from build123d import *

# Parameters (mm, degrees)
F0_W     = 13.3
F0_H     = 13.3
F0_W_2   = 13.4
F0_H_2   = 13.4
F0_W_3   = 13.5
F0_H_3   = 13.5
F0_W_4   = 13.6
F0_H_4   = 13.6
F1_DEPTH = 5


with BuildPart() as f1:
    # F0 (on Top) → F1 (new body)
    with BuildSketch(Plane.XY):
        Polygon((27.294878, 11.65), (-52.963719, 11.65), (-52.963719, -11.65), (30.85, -11.65), (30.85, 8.722694), align=None)
        with Locations((-41.313719, 0)):
            Rectangle(F0_W, F0_H, mode=Mode.SUBTRACT)
        with Locations((-19.05, 0)):
            Rectangle(F0_W_2, F0_H_2, mode=Mode.SUBTRACT)
        Rectangle(F0_W_3, F0_H_3, mode=Mode.SUBTRACT)
        with Locations((19.05, 0)):
            Rectangle(F0_W_4, F0_H_4, mode=Mode.SUBTRACT)
    extrude(amount=F1_DEPTH)


solid = f1.part
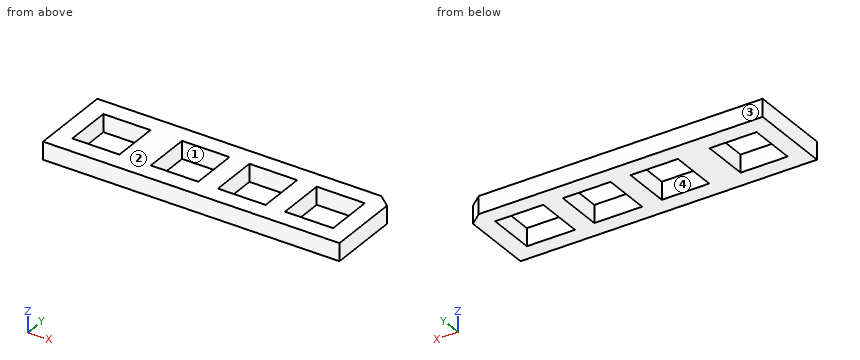
Build history of the part. All positions in model axes, mm. Face numbers are marked on the shaded views. A direction names the side the tool comes from. Round coordinates to 2 decimals unless told otherwise and drop trailing zeros. Loops run counter-clockwise (first coordinate to the right, second up) from the corner with the lowest first, then second, coordinate; pieces in that order, holes last. Notation, with made-up numbers: (-3, 75) -> (34, 75) arc R10 ccw to (34, 94) -> close; hole circle Ø10 at (46, 77.5). An arc over 180 degrees is marked (long way). One line per item, written item: value. Start each with the question number.
Q1. Probe line 1 along X through (y, z) = (-6, 3.3); line 2 along Y through (x, z) = (-19, 4.45); line 3 along Y through (x, z) = (-43, 0.4). List the from-to ranges inside material, lowest first.
Q2. 3-axis set-ups, long thin cutter, end or side, ignore diameter. For the marked faces 1 and 2: which of +Z, -Z, +X, -X, +Y, -Y reach the whole face in a straight line?
Q3. Cut at A-A on x = 23. List the corners of the cut face in (y, z), plus the area to 3 significant figures.
Q4. Cut at B-B on y = 2.75. List the corners of the cut face in (x, z), plus the area to 3 significant figures.
Q5. Two-plate mould, pull along X, no slides. Class the marked faces 3 and 4: released by +X, released by -X, zero draft, split by the parting line, or undercut.
Q6. Cut at C-C on z = 0.95. List the corners of the cut face in (x, y).
Q7. Cut at D-D on x = -18.5. List the corners of the cut face in (y, z).
Computed:
1. line 1: -52.96 to -47.96, -34.66 to -25.75, -12.35 to -6.75, 6.75 to 12.25, 25.85 to 30.85
1. line 2: -11.65 to -6.7, 6.7 to 11.65
1. line 3: -11.65 to -6.65, 6.65 to 11.65
2. face 1: +Z, -Z
2. face 2: +Z, +X, -X, +Y, -Y
3. outline: (-11.65, 0) -> (-6.8, 0) -> (-6.8, 5) -> (-11.65, 5) -> close; (6.8, 0) -> (11.65, 0) -> (11.65, 5) -> (6.8, 5) -> close
3. area: 48.5 mm²
4. outline: (-52.96, 0) -> (-47.96, 0) -> (-47.96, 5) -> (-52.96, 5) -> close; (-34.66, 0) -> (-25.75, 0) -> (-25.75, 5) -> (-34.66, 5) -> close; (-12.35, 0) -> (-6.75, 0) -> (-6.75, 5) -> (-12.35, 5) -> close; (6.75, 0) -> (12.25, 0) -> (12.25, 5) -> (6.75, 5) -> close; (25.85, 0) -> (30.85, 0) -> (30.85, 5) -> (25.85, 5) -> close
4. area: 150 mm²
5. face 3: zero draft
5. face 4: undercut
6. outline: (-52.96, -11.65) -> (30.85, -11.65) -> (30.85, 8.72) -> (27.29, 11.65) -> (-52.96, 11.65) -> close; hole (-47.96, -6.65) -> (-34.66, -6.65) -> (-34.66, 6.65) -> (-47.96, 6.65) -> close; hole (-25.75, -6.7) -> (-12.35, -6.7) -> (-12.35, 6.7) -> (-25.75, 6.7) -> close; hole (-6.75, -6.75) -> (6.75, -6.75) -> (6.75, 6.75) -> (-6.75, 6.75) -> close; hole (12.25, -6.8) -> (25.85, -6.8) -> (25.85, 6.8) -> (12.25, 6.8) -> close
7. outline: (-11.65, 0) -> (-6.7, 0) -> (-6.7, 5) -> (-11.65, 5) -> close; (6.7, 0) -> (11.65, 0) -> (11.65, 5) -> (6.7, 5) -> close
